```python
from build123d import *

# Parameters (mm, degrees)
SKETCH1_R           = 11
BOSS_EXTRUDE1_DEPTH = 3
SKETCH2_R           = 11
SKETCH2_R_2         = 10
BOSS_EXTRUDE2_DEPTH = 3.45
SKETCH4_R           = 5
BOSS_EXTRUDE3_DEPTH = 3.45
SKETCH5_R           = 4
CUT_EXTRUDE1_DEPTH  = 10


with BuildPart() as part:
    # Sketch1 → Boss-Extrude1 (new, symmetric)
    with BuildSketch(Plane(origin=(0, 0, 0), x_dir=(1, 0, 0), z_dir=(0, 1, 0))):
        with Locations(Location((0, 0, 0), (0, 0, 270))):
            Circle(SKETCH1_R)
    extrude(amount=BOSS_EXTRUDE1_DEPTH, both=True)

    # Sketch2 → Boss-Extrude2 (add, symmetric)
    with BuildSketch(Plane(origin=(0, 0, 0), x_dir=(1, 0, 0), z_dir=(0, 1, 0))):
        with Locations(Location((0, 0, 0), (0, 0, 270))):
            Circle(SKETCH2_R)
        with Locations(Location((0, 0, 0), (0, 0, 90))):
            Circle(SKETCH2_R_2, mode=Mode.SUBTRACT)
    extrude(amount=BOSS_EXTRUDE2_DEPTH, both=True)

    # Sketch4 → Boss-Extrude3 (add, symmetric)
    with BuildSketch(Plane(origin=(0, 0, 0), x_dir=(1, 0, 0), z_dir=(0, 1, 0))):
        with Locations(Location((0, 0, 0), (0, 0, 90))):
            Circle(SKETCH4_R)
    extrude(amount=BOSS_EXTRUDE3_DEPTH, both=True)

    # Sketch5 → Cut-Extrude1 (cut)
    with BuildSketch(Plane(origin=(0, 3.45, 0), x_dir=(1, 0, 0), z_dir=(0, 1, 0))):
        with Locations(Location((0, 0, 0), (0, 0, 270))):
            Circle(SKETCH5_R)
    extrude(amount=-CUT_EXTRUDE1_DEPTH, mode=Mode.SUBTRACT)


solid = part.part
```
Verification items for the finished model (mm, model axes). A direction names the side the tool comes from. Round coordinates to 2 decimals unless told otherwise and drop trailing zeros. Loops run counter-clockwise (first coordinate to the right, second up) from the corner with the lowest first, then second, coordinate; pieces in that order, holes last. Notation, with made-up numbers: (-18, 0.25) -> (-14, 0.25) arc R35 cw to (-14, 35.25) -> close; hole circle Ø6 at (78.5, 57.5). An arc over 180 degrees is marked (long way). Answer as a JSON object with one key per item and string values.
Q1. Section check B-B (x = 0). Record the boundary of the cut face in (y, z), then the cut area to 3 significant figures.
Data:
{"outline": "(-3.45, -11) -> (3.45, -11) -> (3.45, -10) -> (3, -10) -> (3, -5) -> (3.45, -5) -> (3.45, -4) -> (-3.45, -4) -> (-3.45, -5) -> (-3, -5) -> (-3, -10) -> (-3.45, -10) -> close; (-3.45, 4) -> (3.45, 4) -> (3.45, 5) -> (3, 5) -> (3, 10) -> (3.45, 10) -> (3.45, 11) -> (-3.45, 11) -> (-3.45, 10) -> (-3, 10) -> (-3, 5) -> (-3.45, 5) -> close", "area": "87.6 mm2"}
Q2. Section check C-C (y = 2.25). Record the boundary of the cut face in (x, z), then the cut area to 3 significant figures.
Data:
{"outline": "circle Ø22 at (0, 0); hole circle Ø8 at (0, 0)", "area": "330 mm2"}
Q3. Section check A-A (z = 0). Record the boundary of the cut face in (x, y), then the cut area to 3 significant figures.
Data:
{"outline": "(-11, -3.45) -> (-10, -3.45) -> (-10, -3) -> (-5, -3) -> (-5, -3.45) -> (-4, -3.45) -> (-4, 3.45) -> (-5, 3.45) -> (-5, 3) -> (-10, 3) -> (-10, 3.45) -> (-11, 3.45) -> close; (4, -3.45) -> (5, -3.45) -> (5, -3) -> (10, -3) -> (10, -3.45) -> (11, -3.45) -> (11, 3.45) -> (10, 3.45) -> (10, 3) -> (5, 3) -> (5, 3.45) -> (4, 3.45) -> close", "area": "87.6 mm2"}
Q4. Scan lines: line 1 (X direction, y = -3.2, z = 0); line 2 (Y direction, x = -9.75, z = -0.25); line 3 (Z direction, x = 2, y = 0). Record each from-to range of solid material in increasing order. Write a range as from..to.
Data:
{"line 1": "x = -11..-10, -5..-4, 4..5, 10..11", "line 2": "y = -3..3", "line 3": "z = -10.82..-3.46, 3.46..10.82"}
Q5. Section check D-D (z = 8.25). Record the boundary of the cut face in (x, y).
Data:
{"outline": "(-7.28, -3.45) -> (-5.65, -3.45) -> (-5.65, -3) -> (5.65, -3) -> (5.65, -3.45) -> (7.28, -3.45) -> (7.28, 3.45) -> (5.65, 3.45) -> (5.65, 3) -> (-5.65, 3) -> (-5.65, 3.45) -> (-7.28, 3.45) -> close"}
Q6. Access from +Z, -Z, +X, -X, +Y, -Y to the whole of each face (thin tool, end or side, straight path). Record for faces 1 (the cylindrical face through (4.88, -3.22, 1.08)), 2 (the cylindrical face through (4.88, 3.23, 1.08)), 3 (the flat face through (-10, 3.45, 2)).
Data:
{"face 1": "-Y", "face 2": "+Y", "face 3": "+Z, -Z, +X, -X, +Y"}
Q7. Draft check along Z on faces 4 (the cylindrical face through (-10.74, 0.05, -2.38)), 5 (the flat face through (-10, -3.45, 2)), 6 (the cylindrical face through (9.76, 3.22, 2.17)). Enter one of: pulls with the +Z half, pulls with the -Z half, needs draft (parallel to the pull), parting line crosses it, or undercut.
Data:
{"face 4": "parting line crosses it", "face 5": "needs draft", "face 6": "undercut"}
